from build123d import *

# Parameters (mm, degrees)
SKETCH1_W           = 51
SKETCH1_H           = 41
SKETCH1_W_2         = 48
SKETCH1_H_2         = 38
BOSS_EXTRUDE1_DEPTH = 1
SKETCH1_3_W         = 51
SKETCH1_3_H         = 41
SKETCH1_3_W_2       = 48
SKETCH1_3_H_2       = 38
BOSS_EXTRUDE2_DEPTH = 10


with BuildPart() as part:
    # Sketch1 → Boss-Extrude1 (new body)
    with BuildSketch(Plane(origin=(0, 0, 0), x_dir=(1, 0, 0), z_dir=(0, 1, 0))):
        Rectangle(SKETCH1_W, SKETCH1_H)
        Rectangle(SKETCH1_W_2, SKETCH1_H_2, mode=Mode.SUBTRACT)
        Rectangle(SKETCH1_W_2, SKETCH1_H_2)
    extrude(amount=BOSS_EXTRUDE1_DEPTH)

    # Sketch1<3> → Boss-Extrude2 (add)
    with BuildSketch(Plane(origin=(0, 0, 0), x_dir=(1, 0, 0), z_dir=(0, 1, 0))):
        Rectangle(SKETCH1_3_W, SKETCH1_3_H)
        Rectangle(SKETCH1_3_W_2, SKETCH1_3_H_2, mode=Mode.SUBTRACT)
    extrude(amount=BOSS_EXTRUDE2_DEPTH)


solid = part.part
Verification items for the finished model (mm, model axes). A direction names the side the tool comes from. Round coordinates to 2 decimals unless told otherwise and drop trailing zeros. Loops run counter-clockwise (first coordinate to the right, second up) from the corner with the lowest first, then second, coordinate; pieces in that order, holes last. Notation, with made-up numbers: (49, 66) - (67, 66) arc R14 ccw to (67, 86) - close; hole circle Ø11 at (-40, 70). An arc over 180 degrees is marked (long way). Use one line per item in the form item = value.
1. Gauge pin test, flat ends, axial feed: pin 1 Ø1.5 at (x, z) = (14.5, 7) entering from +Y; pin 2 Ø8 at (x, z) = (9.5, 5) entering from -Y. Record the tip position at first contact, or that the pin passes through.
A:
pin_1 = 1
pin_2 = 0
2. Draft check along Z on faces 1 (the flat face through (24, 5, 0)), 2 (the flat face through (0, 5, -20.5)), 3 (the flat face through (-2, 10, 20)). Enter one of: pulls with the +Z half, pulls with the -Z half, needs draft (parallel to the pull), parting line crosses it, or undercut.
A:
face_1 = undercut
face_2 = pulls with the -Z half
face_3 = needs draft
3. Access from +Z, -Z, +X, -X, +Y, -Y to the whole of each face (thin tool, end or side, straight path). Record for faces 4 (the flat face through (25.5, 5, 0)), 5 (the flat face through (0, 1, 0)).
A:
face_4 = +Z, -Z, +X, +Y, -Y
face_5 = +Y
4. Scan lines: probe 1 along X at (y, z) = (3.5, 17); probe 2 along Z at (x, y) = (13.5, 2); probe 3 along Y at (x, z) = (3, 8.5). Record each from-to range of solid material in increasing order.
A:
probe_1 = -25.5 to -24, 24 to 25.5
probe_2 = -20.5 to -19, 19 to 20.5
probe_3 = 0 to 1
5. Section check B-B on z = 10. Record the cut outline in (x, y).
A:
outline = (-25.5, 0) - (25.5, 0) - (25.5, 10) - (24, 10) - (24, 1) - (-24, 1) - (-24, 10) - (-25.5, 10) - close
6. Section check A-A on y = 7.75. Record the cut outline in (x, z), and give its area (3 significant figures).
A:
outline = (-25.5, -20.5) - (25.5, -20.5) - (25.5, 20.5) - (-25.5, 20.5) - close; hole (-24, -19) - (24, -19) - (24, 19) - (-24, 19) - close
area = 267 mm²
7. Section check C-C on x = -18. Record the cut outline in (y, z).
A:
outline = (0, -20.5) - (10, -20.5) - (10, -19) - (1, -19) - (1, 19) - (10, 19) - (10, 20.5) - (0, 20.5) - close
